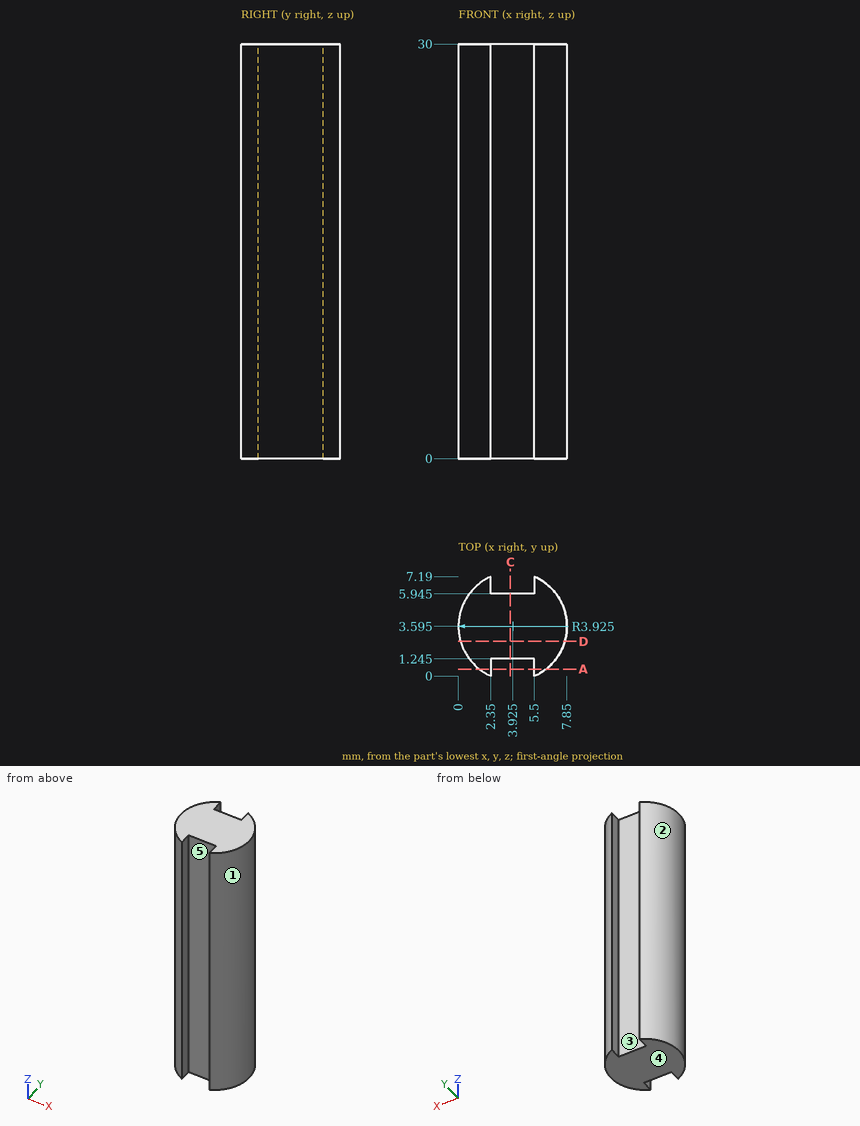
Input: dimensioned drawing with shaded views. Units: mm. Origin: part minimum x, y, z. A direction names the side the tool comes from. Round coordinates to 2 decimals unless told otherwise and drop trailing zeros. Order: outer loops, then holes, each group sorted by start corner. A loop starts at its lowest first (then second) coordinate and runs counter-clockwise, first axis right, second up.
Q1. Pin query (flat end, axial travel): pin 1 (1 mm diameter, centred on y = 7, z = 22, fed in from +X) (1 decimal); pin 2 (1.5 mm diameter, centred on x = 4.5, z = 24.5, fed in from -Y) (3 decimals); pin 3 (0.6 mm diameter, centred on y = 6.5, z = 14.5, fed in from -X). Return the tip coordinate at first contact, or that it passes through.
Result sheet:
pin 1: stops at x = 6.6
pin 2: stops at y = 1.245
pin 3: stops at x = 0.99
Q2. Access query for the marked faces 4 and 5. Directions: +Z, -Z, +X, -X, +Y, -Y. A direction counts if a zero-diameter tool reaches every point of the face in a straight line with its end or side. Return the directions, or none.
Result sheet:
face 4: -Z, +X, -X, +Y, -Y
face 5: +Z, -Z, -Y
Q3. Section C-C, the plane x = 3.75. Output: boundary loops of the cut face in (y, z) (1 decimal).
Result sheet:
outline: (1.2, 0) - (5.9, 0) - (5.9, 30) - (1.2, 30) - close
Q4. Material intervals for probe 1 along Y at (x, z) = (5, 17) (1 decimal); probe 2 along X at (y, z) = (0.5, 24); probe 3 along X at (y, z) = (3.5, 2.75), sorted ascending.
Result sheet:
probe 1: y = 1.2 to 5.9
probe 2: x = 1.51 to 2.35, 5.5 to 6.34
probe 3: x = 0 to 7.85
Q5. Section A-A, the plane y = 0.5. Output: boundary loops of the cut face in (x, z).
Result sheet:
outline: (1.51, 0) - (2.35, 0) - (2.35, 30) - (1.51, 30) - close; (5.5, 0) - (6.34, 0) - (6.34, 30) - (5.5, 30) - close
Q6. Section D-D, the plane y = 2.5. Output: boundary loops of the cut face in (x, z), and give its area (3 significant figures).
Result sheet:
outline: (0.16, 0) - (7.69, 0) - (7.69, 30) - (0.16, 30) - close
area: 226 mm2
Q7. Mould query, pull axis X, two halves, no side actions, for the marked faces 1, 2 and 3. Classes: released by +X, released by -X, zero draft, split by the parting line, or undercut.
Result sheet:
face 1: released by +X
face 2: released by -X
face 3: undercut
